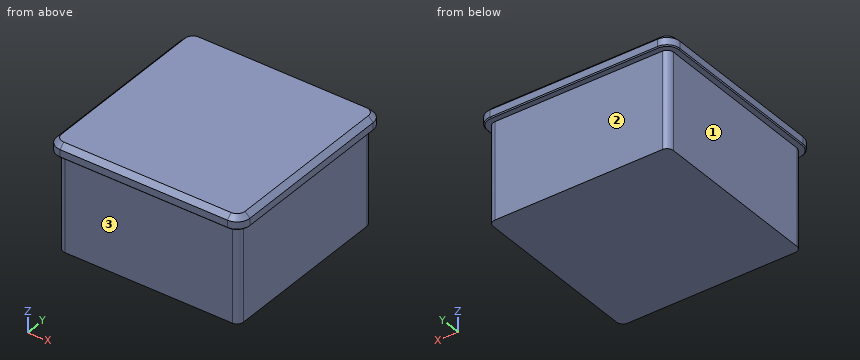
Autodesk Inventor part; units mm, degrees
ref_plane "YZ Plane" through (0, 0, 0) normal (1, 0, 0) x (0, 1, 0)
ref_plane "XZ Plane" through (0, 0, 0) normal (0, 1, 0) x (-1, 0, 0)
ref_plane "XY Plane" through (0, 0, 0) normal (0, 0, 1) x (1, 0, 0)
sketch "Sketch1" plane through (0, 0, 0) normal (0, 0, 1) x (1, 0, 0)
  line L0 (26, 23) -> (-26, 23)
  arc A0 (-26, 23) -> (-28, 21) centre (-26, 21) ccw
  line L1 (-28, 21) -> (-28, -31)
  arc A1 (28, 21) -> (26, 23) centre (26, 21) ccw
  line L2 (28, -31) -> (28, 21)
  arc A2 (26, -33) -> (28, -31) centre (26, -31) ccw
  line L3 (-26, -33) -> (26, -33)
  arc A3 (-28, -31) -> (-26, -33) centre (-26, -31) ccw
  point P0 (0, 0)
extrude "Extrusion1" add sketch "Sketch1" against normal blind 30
sketch "Sketch2" plane through (0, 0, 0) normal (0, 0, 1) x (1, 0, 0)
  line L0 (26, 23) -> (-26, 23)
  arc A0 (28, 21) -> (26, 23) centre (26, 21) ccw
  line L1 (28, -31) -> (28, 21)
  arc A1 (26, -33) -> (28, -31) centre (26, -31) ccw
  line L2 (-26, -33) -> (26, -33)
  arc A2 (-28, -31) -> (-26, -33) centre (-26, -31) ccw
  line L3 (-28, 21) -> (-28, -31)
  arc A3 (-26, 23) -> (-28, 21) centre (-26, 21) ccw
  line L4 (-30, -31) -> (-30, 21)
  arc A4 (-30, -31) -> (-26, -35) centre (-26, -31) ccw
  line L5 (26, -35) -> (-26, -35)
  arc A5 (26, -35) -> (30, -31) centre (26, -31) ccw
  line L6 (30, 21) -> (30, -31)
  arc A6 (30, 21) -> (26, 25) centre (26, 21) ccw
  line L7 (-26, 25) -> (26, 25)
  arc A7 (-26, 25) -> (-30, 21) centre (-26, 21) ccw
  point P0 (0, 0)
extrude "Extrusion2" add sketch "Sketch2" along normal blind 4 contours A0 L1 A1 L2 A2 L3 A3 L0 | L4 A7 L7 A6 L6 A5 L5 A4
chamfer "Chamfer1" distance 1.5 angle 45 8 edges at (-30, -5, 4) (-28.8284, -33.8284, 4) (0, -35, 4) (28.8284, -33.8284, 4) (30, -5, 4) (28.8284, 23.8284, 4) (0, 25, 4) (-28.8284, 23.8284, 4)
chamfer "Chamfer2" distance 0.3 angle 45 8 edges at (-30, -5, 0) (-28.8284, 23.8284, 0) (0, 25, 0) (28.8284, 23.8284, 0) (30, -5, 0) (28.8284, -33.8284, 0) (0, -35, 0) (-28.8284, -33.8284, 0)
properties part number "nút nhựa bịt hộp thép 60x60"
Geometry check sheet. Reference: the model listing, model coordinates, mm. Face numbers are marked on the shaded views. A direction names the side the tool comes from. Round coordinates to 2 decimals unless told otherwise and drop trailing zeros. Loops run counter-clockwise (first coordinate to the right, second up) from the corner with the lowest first, then second, coordinate; pieces in that order, holes last. Notation, with made-up numbers: (-36.5, 82) -> (-7.5, 82) arc R25 ccw to (-7.5, 102) -> close; hole circle Ø3 at (30.25, 89.5). An arc over 180 degrees is marked (long way). Answer as a JSON object with one key per item and string values. Group by question number.
Item 1: Depth check by flat-ended pin: pin 1 Ø1 at (y, z) = (-15.5, -23.5) entering from -X; pin 2 Ø4 at (x, z) = (1, -13.5) entering from -Y; pin 3 Ø8 at (x, z) = (-5.5, -17) entering from +Y; pin 4 Ø12 at (y, z) = (-10, -4) entering from +X. Enter the tip coordinate at first touch or a pass-through.
Item 2: Cross-section at C-C, the plane x = 10. Record the cut outline in (y, z).
Item 3: Cross-section at B-B, the plane z = -10.5. Record the cut outline in (x, y), plus the area to 3 significant figures.
Item 4: Cross-section at A-A, the plane y = -2.5. Record the cut outline in (x, z).
Item 5: Set-up check for the marked faces 1, 2 and 3: record each of +Z, -Z, +X, -X, +Y, -Y from which the full face is reachable in a straight line by a thin tool's end or side.
Item 6: Thickness scan on line 1 along X through (y, z) = (-18, -11.5); line 2 along Y through (x, z) = (5, -1); line 3 along X through (y, z) = (22, -25). Record the ranges inside material, lowest first.
Determined:
{
 "1": {"pin 1": "stops at x = -28", "pin 2": "stops at y = -33", "pin 3": "stops at y = 23", "pin 4": "stops at x = 30"},
 "2": {"outline": "(-35, 0.3) -> (-34.7, 0) -> (-33, 0) -> (-33, -30) -> (23, -30) -> (23, 0) -> (24.7, 0) -> (25, 0.3) -> (25, 2.5) -> (23.5, 4) -> (-33.5, 4) -> (-35, 2.5) -> close"},
 "3": {"outline": "(-28, -31) arc R2 ccw to (-26, -33) -> (26, -33) arc R2 ccw to (28, -31) -> (28, 21) arc R2 ccw to (26, 23) -> (-26, 23) arc R2 ccw to (-28, 21) -> close", "area": "3,130 mm²"},
 "4": {"outline": "(-30, 0.3) -> (-29.7, 0) -> (-28, 0) -> (-28, -30) -> (28, -30) -> (28, 0) -> (29.7, 0) -> (30, 0.3) -> (30, 2.5) -> (28.5, 4) -> (-28.5, 4) -> (-30, 2.5) -> close"},
 "5": {"face 1": "-Z, -X, +Y, -Y", "face 2": "-Z, +X, -X, +Y", "face 3": "-Z, +X, -X, -Y"},
 "6": {"line 1": "x = -28 to 28", "line 2": "y = -33 to 23", "line 3": "x = -27.73 to 27.73"}
}
